```python
from build123d import *

# Parameters (mm, degrees)
REVOLU_O1_ANGLE          = 180
RESSALTO_EXTRUS_O1_DEPTH = 2
ESBO_O7_R                = 2.5
CORTE_EXTRUS_O1_DEPTH    = 29.0000001
ESBO_O8_R                = 2
CORTE_EXTRUS_O2_DEPTH    = 29.0000001


with BuildPart() as part:
    # Varredura1: sweep along a path in Esboço1
    with BuildLine(Plane.XY) as varredura1_path:
        ThreePointArc((0, 0), (16.529462147, 0.705444386), (33, 2.268183475))
        ThreePointArc((33, 2.268183475), (58.050044629, 5.646181244), (83, 9.697765111))
        ThreePointArc((83, 9.697765111), (93.959586917, 11.235067223), (105, 12))
    # Esboço2 → Varredura1 (sweep)
    with BuildSketch(Plane(origin=(0, 0, 0), x_dir=(0, 0, -1), z_dir=(1, 0, 0))):
        with BuildLine():
            Line((-14, 7.442730927), (-14, 0.894376808))
            ThreePointArc((-14, 0.894376808), (-13.5, 0.394376808), (-13, 0.894376808))
            Line((-13, 0.894376808), (-13, 6.736019744))
            ThreePointArc((-13, 6.736019744), (-12.74508542, 7.380356175), (-12.118337614, 7.675886319))
            ThreePointArc((-12.118337614, 7.675886319), (-6.062261288, 7.966491733), (0, 8.063959997))
            ThreePointArc((0, 8.063959997), (6.062261288, 7.966491733), (12.118337614, 7.675886319))
            ThreePointArc((12.118337614, 7.675886319), (12.74508542, 7.380356175), (13, 6.736019744))
            Line((13, 6.736019744), (13, 0.894376808))
            ThreePointArc((13, 0.894376808), (13.5, 0.394376808), (14, 0.894376808))
            Line((14, 0.894376808), (14, 7.442730927))
            ThreePointArc((14, 7.442730927), (13.576954157, 8.486842866), (12.546440343, 8.942011852))
            ThreePointArc((12.546440343, 8.942011852), (0, 9.136278747), (-12.546440343, 8.942011852))
            ThreePointArc((-12.546440343, 8.942011852), (-13.576954157, 8.486842866), (-14, 7.442730927))
        make_face()
    sweep(path=varredura1_path.line)

    # Esboço3 → Revolução1 (revolve)
    with BuildSketch(Plane(origin=(105.176984905, 1.830436311, 0), x_dir=(0, 0, -1), z_dir=(0.999848595, 0.017400757, 0))):
        with BuildLine():
            Line((14, 17.613834568), (14, 11.065480449))
            ThreePointArc((14, 11.065480449), (13.5, 10.565480449), (13, 11.065480449))
            Line((13, 11.065480449), (13, 16.907123386))
            ThreePointArc((13, 16.907123386), (12.74508542, 17.551459816), (12.118337614, 17.84698996))
            ThreePointArc((12.118337614, 17.84698996), (6.062261288, 18.137595374), (0, 18.235063639))
            Line((0, 18.235063639), (0, 19.307382388))
            ThreePointArc((0, 19.307382388), (6.273972125, 19.258812754), (12.546440343, 19.113115494))
            ThreePointArc((12.546440343, 19.113115494), (13.576954157, 18.657946508), (14, 17.613834568))
        make_face()
    revolve(axis=Axis((104.841021832, 21.134895472, 0), (0.017400757, -0.999848595, 0)), revolution_arc=REVOLU_O1_ANGLE)

    # Esboço6 → Ressalto-extrusão1 (add)
    with BuildSketch(Plane.XY.offset(14)):
        with BuildLine():
            Line((0, 7.442730927), (-7, -4.557269073))
            Line((-7, -4.557269073), (-5.272442198, -5.565011124))
            ThreePointArc((-5.272442198, -5.565011124), (-0.943881137, -10.614607271), (3.685022716, -5.838823437))
            Line((3.685022716, -5.838823437), (27.464771889, -6.644799062))
            ThreePointArc((27.464771889, -6.644799062), (29.011913143, -6.198294277), (29.999382133, -4.926320387))
            Line((29.999382133, -4.926320387), (32.907249231, 3.157737954))
            Line((32.907249231, 3.157737954), (32.2281564, 9.670784444))
            ThreePointArc((32.2281564, 9.670784444), (16.14315941, 8.136106307), (0, 7.442730927))
        make_face()
    ressalto_extrus_o1 = extrude(amount=-RESSALTO_EXTRUS_O1_DEPTH)

    # Espelhar1: Ressalto-extrusão1 across plane
    add(ressalto_extrus_o1.mirror(Plane.XY))

    # Esboço7 → Corte-extrusão1 (cut, through all)
    with BuildSketch(Plane.XY.offset(14)):
        with Locations((-0.806389095, -6.116708213)):
            Circle(ESBO_O7_R)
    extrude(amount=-CORTE_EXTRUS_O1_DEPTH, mode=Mode.SUBTRACT)

    # Esboço8 → Corte-extrusão2 (cut, through all)
    with BuildSketch(Plane.XY.offset(14)):
        with Locations((25.307249231, -3.369835879)):
            Circle(ESBO_O8_R)
    extrude(amount=-CORTE_EXTRUS_O2_DEPTH, mode=Mode.SUBTRACT)


solid = part.part
```
Read the model definition and answer for the solid it produces. Units are mm, in the model's axes. A direction names the side the tool comes from. Coordinates: 2 decimals unless noted, no trailing zeros. Order: outer loops, then holes, each group sorted by start corner. A loop starts at its lowest first (then second) coordinate and runs counter-clockwise, first axis right, second up. Notation, with made-up numbers: (-22, 59.25) - (-10, 59.25) arc R14 cw to (-10, 83.25) - close; hole circle Ø3 at (58.5, 6). An arc over 180 degrees is marked (long way). Answer as a JSON object with one key per item and string values. Group by question number.
Item 1: Flat-ended cylindrical pins translate along their axes: P1, Ø12, axis at x = 32, z = 9.5, coming from the +Y side; P2, Ø4, axis at x = 17.5, z = -4, coming from the -Y side; P3, Ø3, axis at x = 52, z = 6.5, coming from the +Y side. Find the tip coordinate at first contact, or state that the pin passes through.
Item 2: The mould has two halves that part along Z. Classify faces 1 (the face through (28.993, -6.211, -13.014)), 2 (the face through (68, 11, 13)), 3 (the face through (118.923, 16.366, -0.308)), 4 (the face through (40, 6, 14)): +Z half, -Z half, draft (parallel to the pull), parting line (faces both ways), or undercut.
Item 3: Consider probe 1 along Z at (x, y) = (15, 0.5); probe 2 along Z at (x, y) = (83, 12.5); probe 3 along Y at (x, z) = (108, 1.5). Determine where each line is inside the solid, lowest interval first. Write a range as from..to.
Item 4: Section A-A (y = 0) is taken. Give the vertices of the cut face in (x, z), plus the area to 3 significant figures.
Item 5: A tool of negligible diameter and unlimited length cuts with its end or side. For faces 5 (the face through (117.928, 16.082, -0.286)), 6 (the face through (27.215, -2.769, -12.986)), 7 (the face through (16.37, 8.15, -12.35)), from which of +Z, -Z, +X, -X, +Y, -Y can it reach the whole face along a straight path? Write none if from no direction.
Results are:
{
 "1": {"P1": "stops at y = 12", "P2": "stops at y = 8.67", "P3": "stops at y = 14.16"},
 "2": {"face 1": "draft", "face 2": "undercut", "face 3": "parting line", "face 4": "+Z half"},
 "3": {"probe 1": "z = -14..-12, 12..14", "probe 2": "z = -14..-13, 13..14", "probe 3": "y = 20.09..21.17"},
 "4": {"outline": "(-4.34, -14) - (31.77, -14) - (31.77, -12) - (-4.34, -12) - close; (-4.34, 12) - (31.77, 12) - (31.77, 14) - (-4.34, 14) - close", "area": "144 mm^2"},
 "5": {"face 5": "-Y", "face 6": "+Z, -Z", "face 7": "none"}
}
